from build123d import *

# Parameters (mm, degrees)
SKETCH1_W                      = 160
SKETCH1_H                      = 60
BOSS_EXTRUDE1_DEPTH            = 4
M3_CLEARANCE_HOLE1_D           = 3.4
M3_CLEARANCE_HOLE1_CSINK_D     = 3.45
M3_CLEARANCE_HOLE1_CSINK_ANGLE = 90


with BuildPart() as part:
    # Sketch1 → Boss-Extrude1 (new body)
    with BuildSketch(Plane(origin=(0, 0, 0), x_dir=(1, 0, 0), z_dir=(0, 1, 0))):
        with Locations((80, 30)):
            Rectangle(SKETCH1_W, SKETCH1_H)
    extrude(amount=BOSS_EXTRUDE1_DEPTH)

    # M3 Clearance Hole1 (through all)
    with Locations(Plane(origin=(0, 4, 0), x_dir=(1, 0, 0), z_dir=(0, 1, 0))):
        with Locations((155, 55), (5, 5), (55, 5), (105, 5), (155, 5), (5, 55), (55, 55), (105, 55)):
            CounterSinkHole(M3_CLEARANCE_HOLE1_D / 2, M3_CLEARANCE_HOLE1_CSINK_D / 2, counter_sink_angle=M3_CLEARANCE_HOLE1_CSINK_ANGLE)


solid = part.part
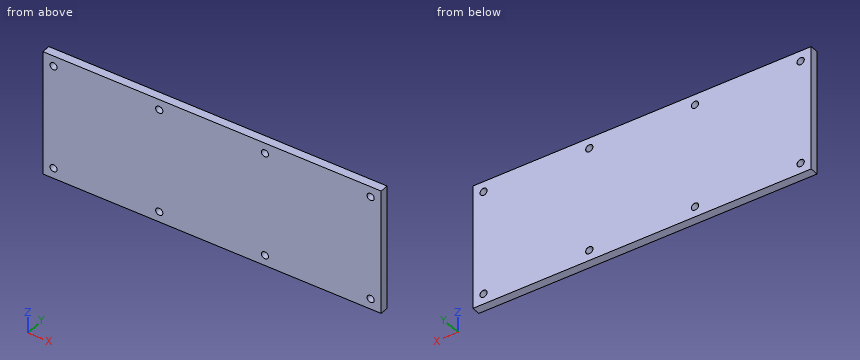
For this review, take the finished solid that the model builds, in its own axes (mm). Give positions to 0.01 mm unless a question says otherwise; leave off trailing zeros. Loops run counter-clockwise (first coordinate to the right, second up) from the corner with the lowest first, then second, coordinate; pieces in that order, holes last.
Item 1: Take a section at B-B, the plane z = -55. State the section outline as (x, y) points (3 decimals), and give its area (3 significant figures).
Item 2: Take a section at A-A, the plane x = 155. State the section outline as (y, z) points (3 decimals), and give its area (3 significant figures).
Item 3: For line 1 along Z through (x, y) = (105, 1.75); line 2 along X through (y, z) = (1.55, -5); line 3 along X through (y, z) = (1.05, -54.5), list the stretches that pass through material, from the lowest coordinate up.
Calculated:
1. outline: (0, 0) - (3.3, 0) - (3.3, 3.975) - (3.275, 4) - (0, 4) - close; (6.7, 0) - (53.3, 0) - (53.3, 3.975) - (53.275, 4) - (6.725, 4) - (6.7, 3.975) - close; (56.7, 0) - (103.3, 0) - (103.3, 3.975) - (103.275, 4) - (56.725, 4) - (56.7, 3.975) - close; (106.7, 0) - (153.3, 0) - (153.3, 3.975) - (153.275, 4) - (106.725, 4) - (106.7, 3.975) - close; (156.7, 0) - (160, 0) - (160, 4) - (156.725, 4) - (156.7, 3.975) - close
1. area: 586 mm2
2. outline: (0, -60) - (4, -60) - (4, -56.725) - (3.975, -56.7) - (0, -56.7) - close; (0, -53.3) - (3.975, -53.3) - (4, -53.275) - (4, -6.725) - (3.975, -6.7) - (0, -6.7) - close; (0, -3.3) - (3.975, -3.3) - (4, -3.275) - (4, 0) - (0, 0) - close
2. area: 213 mm2
3. line 1: z = -60 to -56.7, -53.3 to -6.7, -3.3 to 0
3. line 2: x = 0 to 3.3, 6.7 to 53.3, 56.7 to 103.3, 106.7 to 153.3, 156.7 to 160
3. line 3: x = 0 to 3.38, 6.62 to 53.38, 56.62 to 103.38, 106.62 to 153.38, 156.62 to 160
